from build123d import *

# Parameters (mm, degrees)
SKETCH2_R                           = 4.953
SKETCH2_R_2                         = 2.413
BOSS_EXTRUDE1_DEPTH                 = 8.89
BOSS_EXTRUDE2_START                 = 4.7625
SKETCH2_2_R                         = 4.953
SKETCH2_2_R_2                       = 2.413
SKETCH2_2_R_3                       = 1.9939
BOSS_EXTRUDE2_DEPTH                 = 4.7625
CUT_EXTRUDE1_REACH                  = 13.318
CUT_EXTRUDE1_END_RADIUS             = 4.953
SKETCH8_R                           = 1.411111111
CUT_EXTRUDE1_DIRECTION_2_REACH      = 13.318
CUT_EXTRUDE1_DIRECTION_2_END_RADIUS = 4.953
FILLET2_R                           = 1.27


with BuildPart() as part:
    # Sketch2 → Boss-Extrude1 (new body)
    with BuildSketch(Plane.XY):
        Circle(SKETCH2_R)
        Circle(SKETCH2_R_2, mode=Mode.SUBTRACT)
    extrude(amount=-BOSS_EXTRUDE1_DEPTH)

    # Sketch2<2> → Boss-Extrude2 (add)
    # profile 1 of 3: a face of its own
    with BuildSketch(Plane.XY.offset(BOSS_EXTRUDE2_START)):
        Circle(SKETCH2_2_R)
        Circle(SKETCH2_2_R_2, mode=Mode.SUBTRACT)
    # profile 2 of 3: a face of its own
    with BuildSketch(Plane.XY.offset(BOSS_EXTRUDE2_START)):
        Circle(SKETCH2_2_R_2)
        Circle(SKETCH2_2_R_3, mode=Mode.SUBTRACT)
    # profile 3 of 3: a face of its own
    with BuildSketch(Plane.XY.offset(BOSS_EXTRUDE2_START)):
        Circle(SKETCH2_2_R_3)
    extrude(amount=-BOSS_EXTRUDE2_DEPTH)

    # Cut-Extrude1: up to this cylinder (the profile starts inside it)
    cut_extrude1_end = Plane(origin=(0, 0, 2.54), z_dir=(0, 0, 1)) * Cylinder(CUT_EXTRUDE1_END_RADIUS, 37.542, mode=Mode.PRIVATE)
    # Sketch8 → Cut-Extrude1 (cut, up to the surface)
    with BuildSketch(Plane(origin=(0, 0, 0), x_dir=(1, 0, 0), z_dir=(0, 1, 0)), mode=Mode.PRIVATE) as cut_extrude1_sk1:
        with Locations(Location((0, -2.54, 0), (0, 0, 90))):
            Circle(SKETCH8_R)
    cut_extrude1_tool1 = extrude(cut_extrude1_sk1.sketch, amount=-CUT_EXTRUDE1_REACH, mode=Mode.PRIVATE) & cut_extrude1_end
    add(cut_extrude1_tool1.solids().sort_by_distance((0, 0, 2.54))[0], mode=Mode.SUBTRACT)

    # Cut-Extrude1 direction 2: up to this cylinder (the profile starts inside it)
    cut_extrude1_direction_2_end = Plane(origin=(0, 0, 2.54), z_dir=(0, 0, 1)) * Cylinder(CUT_EXTRUDE1_DIRECTION_2_END_RADIUS, 37.542, mode=Mode.PRIVATE)
    # Sketch8 → Cut-Extrude1 direction 2 (cut, up to the surface)
    with BuildSketch(Plane(origin=(0, 0, 0), x_dir=(1, 0, 0), z_dir=(0, 1, 0)), mode=Mode.PRIVATE) as cut_extrude1_direction_2_sk1:
        with Locations(Location((0, -2.54, 0), (0, 0, 90))):
            Circle(SKETCH8_R)
    cut_extrude1_direction_2_tool1 = extrude(cut_extrude1_direction_2_sk1.sketch, amount=CUT_EXTRUDE1_DIRECTION_2_REACH, mode=Mode.PRIVATE) & cut_extrude1_direction_2_end
    add(cut_extrude1_direction_2_tool1.solids().sort_by_distance((0, 0, 2.54))[0], mode=Mode.SUBTRACT)

    # Fillet2
    # the kernel refuses this fillet: 1.27 mm, written as the material it takes off along each edge
    with BuildSketch(Plane(origin=(0, 0, -8.89), x_dir=(1, 0, 0), z_dir=(0, -1, 0))) as fillet2_piece_1:
        with BuildLine():
            CenterArc((4.953 - FILLET2_R, FILLET2_R), FILLET2_R, 270, 90)
            Line((4.953 - FILLET2_R, 0), (4.953, 0))
            Line((4.953, 0), (4.953, FILLET2_R))
        make_face()
    revolve(axis=Axis((0, 0, -8.89), (0, 0, 1)), mode=Mode.SUBTRACT)
    with BuildSketch(Plane(origin=(0, 0, 4.7625), x_dir=(1, 0, 0), z_dir=(0, -1, 0))) as fillet2_piece_2:
        with BuildLine():
            CenterArc((4.953 - FILLET2_R, -FILLET2_R), FILLET2_R, 0, 90)
            Line((4.953 - FILLET2_R, 0), (4.953, 0))
            Line((4.953, 0), (4.953, -FILLET2_R))
        make_face()
    revolve(axis=Axis((0, 0, 4.7625), (0, 0, 1)), mode=Mode.SUBTRACT)


solid = part.part
Can you work these out from the model? Positions are in its coordinate system, mm. A direction names the side the tool comes from. Give positions to 0.01 mm unless a question says otherwise; leave off trailing zeros. Order: outer loops, then holes, each group sorted by start corner. A loop starts at its lowest first (then second) coordinate and runs counter-clockwise, first axis right, second up. Notation, with made-up numbers: M 9,-39 L 37,-39 A19 ccw 37,-26 Z; hole C 24,67 d5. An arc over 180 degrees is marked long. One line per question, with ' | ' between items.
Item 1: I'm going to push flat-ended pins straight in: pin 1 Ø1 at (x, z) = (-3, -0.5) entering from +Y; pin 2 Ø3 at (x, y) = (2.5, 3.5) entering from +Z; pin 3 Ø4 at (y, z) = (3.5, -5) entering from +X; pin 4 Ø1 at (x, z) = (4, -4) entering from -Y. Where does each tip first touch, or does it pass through?
Answer block:
pin 1: stops at y = 4.28 | pin 2: stops at z = 4.76 | pin 3: stops at x = 4.72 | pin 4: stops at y = -3.5
Item 2: Suppose I cut it at C-C, the plane z = -5.75. Write out the boundary of the cut face in (x, y), then the cut area to 3 significant figures.
Answer block:
outline: C 0,0 d9.91; hole C 0,0 d4.83 | area: 58.8 mm2
Item 3: Suppose I cut it at A-A, the plane y = 0. Write out the boundary of the cut face in (x, z).
Answer block:
outline: M -4.95,-7.62 A1.27 ccw -3.68,-8.89 L -2.41,-8.89 L -2.41,0 L 2.41,0 L 2.41,-8.89 L 3.68,-8.89 A1.27 ccw 4.95,-7.62 L 4.95,3.49 A1.27 ccw 3.68,4.76 L -3.68,4.76 A1.27 ccw -4.95,3.49 Z; hole C 0,2.54 d2.82
Item 4: Suppose I cut it at B-B, the plane x = 0. Write out the boundary of the cut face in (y, z).
Answer block:
outline: M -4.95,-7.62 A1.27 ccw -3.68,-8.89 L -2.41,-8.89 L -2.41,0 L 2.41,0 L 2.41,-8.89 L 3.68,-8.89 A1.27 ccw 4.95,-7.62 L 4.95,1.13 L -4.95,1.13 Z; M -4.87,3.95 L 4.87,3.95 A1.27 ccw 3.68,4.76 L -3.68,4.76 A1.27 ccw Z
Item 5: Suppose I cut it at D-D, the plane z = 2.54. Write out the boundary of the cut face in (x, y), then the cut area to 3 significant figures.
Answer block:
outline: M -1.41,-4.75 L -1.41,4.75 A4.95 ccw Z; M 1.41,-4.75 A4.95 ccw 1.41,4.75 Z | area: 49.5 mm2
Item 6: Please list where these lines run through material, in increasing order: L1, parallel to Y at x = 0, z = -7; L2, parallel to X at y = 0.5, z = 2.54; L3, parallel to X at y = 3, z = 1.75.
Answer block:
L1: y = -4.95 to -2.41, 2.41 to 4.95 | L2: x = -4.93 to -1.41, 1.41 to 4.93 | L3: x = -3.94 to -1.17, 1.17 to 3.94
Item 7: We'd pull the mould along Y, two halves only. Please class faces 1 (the face through (-0.06, 0.07, 3.95)), 2 (the face through (-1.915, -1.468, -4.383)), 3 (the face through (4.724, 1.488, -1.986)): released by +Y, released by -Y, zero draft, split by the parting line, or undercut.
Answer block:
face 1: zero draft | face 2: undercut | face 3: split by the parting line
Item 8: For faces 4 (the face through (0, 0, 4.762)), 5 (the face through (0, 0, 0)), which set-ups out of +Z, -Z, +X, -X, +Y, -Y let a thin tool reach every point of the face, with its end or its side?
Answer block:
face 4: +Z, +X, -X, +Y, -Y | face 5: -Z
